Could you check a few things on this model? Use its own coordinates, in mm. A direction names the side the tool comes from. Give positions to 0.01 mm unless a question says otherwise; leave off trailing zeros. Write each loop counter-clockwise with the first axis right and the second up, starting at its lowest first coordinate (ties: lowest second). Pieces come first, ordered by that corner, then holes. Notation, with made-up numbers: M 34.25,9 L 90.25,9 A24 ccw 90.25,24 Z; hole C 26.25,-22 d7. An arc over 180 degrees is marked long. Use one line per item in the form item = value.
from build123d import *

# Parameters (mm, degrees)
PAD_DEPTH             = 12.6
SKETCH001_R           = 3.6
POCKET_DEPTH          = 12.601
FILLET_R              = 7
CLONE_PLACEMENT_ANGLE = 180


with BuildPart() as part:
    # Sketch → Pad (new body)
    with BuildSketch(Plane.XY):
        with BuildLine():
            Line((0, 0), (0, -74.09))
            Line((0, -74.09), (-40.005, -74.09))
            Line((-40.005, -74.09), (-40.005, -32))
            ThreePointArc((-40.005, -32), (-41.938095, -27.333095), (-46.605, -25.4))
            Line((-46.605, -25.4), (-81.28, -25.4))
            Line((-81.28, -25.4), (-81.28, 0))
            Line((-81.28, 0), (0, 0))
        make_face()
    extrude(amount=PAD_DEPTH)

    # Sketch001 (on Face9 of Pad) → Pocket (cut, through all)
    with BuildSketch(Plane.XY.offset(12.6)):
        with Locations((-73.9775, -6.35)):
            Circle(SKETCH001_R)
        with Locations((-7.9375, -6.35)):
            Circle(SKETCH001_R)
        with Locations((-40.9575, -6.35)):
            Circle(SKETCH001_R)
        with Locations((-28.575, -31.75)):
            Circle(SKETCH001_R)
        with Locations((-9.525, -31.75)):
            Circle(SKETCH001_R)
        with Locations((-28.575, -49.75)):
            Circle(SKETCH001_R)
        with Locations((-9.525, -49.75)):
            Circle(SKETCH001_R)
        with Locations((-28.575, -67.75)):
            Circle(SKETCH001_R)
        with Locations((-9.525, -67.75)):
            Circle(SKETCH001_R)
    extrude(amount=-POCKET_DEPTH, mode=Mode.SUBTRACT)

    # Fillet
    fillet_edges = [part.edges().sort_by_distance(p)[0] for p in [
        (0, 0, 6.3),
        (-81.28, 0, 6.3),
        (-81.28, -25.4, 6.3),
        (-40.005, -74.09, 6.3),
        (0, -74.09, 6.3),
    ]]
    fillet(fillet_edges, radius=FILLET_R)


with BuildPart() as part_1:
    # Clone placement: moved
    add(part.part.moved(Location((0, 0, -12.6))).rotate(Axis((0, 0, -12.6), (0, 0, 1)), CLONE_PLACEMENT_ANGLE))


solid = part_1.part
1) I want a section at D-D, the plane x = 42. Please give me the cut outline in (y, z).
Checked values:
outline = M 0,-12.6 L 2.9,-12.6 L 2.9,0 L 0,0 Z; M 9.8,-12.6 L 27.27,-12.6 L 27.27,0 L 9.8,0 Z
2) If I drill on L1, parallel to Y at x = 28.5, z = -10.25; L2, parallel to X at y = 64.5, z = -9.75 (3 decimals); L3, parallel to X at y = 31.75, z = -5 (3 decimals), over which ranges is the centre line in solid material (lowest first)?
Checked values:
L1 = 0 to 28.15, 35.35 to 46.15, 53.35 to 64.15, 71.35 to 74.09
L2 = 0 to 7.977, 11.073 to 27.027, 30.123 to 40.005
L3 = 0 to 5.925, 13.125 to 24.975, 32.175 to 40.01
3) For faces 5 (the cylindrical face through (72.316, 9.544, -6.212)), 6 (the flat face through (60, 25.4, -6)), which set-ups out of +Z, -Z, +X, -X, +Y, -Y let a thin tool reach every point of the face, with its end or its side?
Checked values:
face_5 = +Z, -Z
face_6 = +Z, -Z, +X, +Y
4) Thinking about a two-plate mould opening in X: for faces 1 (the flat face through (0, 37, -6)), 2 (the flat face through (31, 28, 0)), 3 (the cylindrical face through (31.23, 29.32, -6.21)), 4 (the cylindrical face through (79.28, 23.3, -6.21)), which applies, released by +X, released by -X, zero draft, split by the parting line, or undercut?
Checked values:
face_1 = released by -X
face_2 = zero draft
face_3 = undercut
face_4 = released by +X
5) I want a section at C-C, the plane y = 30. Please give me the cut outline in (x, z), plus the area to 3 significant figures.
Checked values:
outline = M 0,-12.6 L 6.38,-12.6 L 6.38,0 L 0,0 Z; M 12.67,-12.6 L 25.43,-12.6 L 25.43,0 L 12.67,0 Z; M 31.72,-12.6 L 40.32,-12.6 L 40.32,0 L 31.72,0 Z
area = 349 mm2
6) For pin 1 Ø4 at (x, z) = (66.5, -3.5) entering from +Y, with a flat end and sliding along its axis, tell me the tip position at first contact or that it passes through.
Checked values:
pin_1 = 25.4
7) I want a section at B-B, the plane x = 29.5. Please give me the cut outline in (y, z).
Checked values:
outline = M 0,-12.6 L 28.27,-12.6 L 28.27,0 L 0,0 Z; M 35.23,-12.6 L 46.27,-12.6 L 46.27,0 L 35.23,0 Z; M 53.23,-12.6 L 64.27,-12.6 L 64.27,0 L 53.23,0 Z; M 71.23,-12.6 L 74.09,-12.6 L 74.09,0 L 71.23,0 Z
8) I want a section at A-A, the plane z = -5.25. Count the separate pieces of the cut face and the enclosed holes in it, plus the area to 3 significant figures.
Checked values:
separate_pieces = 1
enclosed_holes = 9
area = 3,600 mm2
